```python
from build123d import *

# Parameters (mm, degrees)
BOSS_EXTRUDE1_DEPTH = 8
SKETCH12_W          = 1.5
SKETCH12_H          = 8.6
BOSS_EXTRUDE8_DEPTH = 3
BOSS_EXTRUDE5_DEPTH = 3
BOSS_EXTRUDE6_START = 8.75
SKETCH10_R          = 1.75
BOSS_EXTRUDE6_DEPTH = 8.75
SKETCH11_W          = 14.1
SKETCH11_H          = 1.5
BOSS_EXTRUDE7_DEPTH = 1.5
FILLET1_R           = 2
CUT_EXTRUDE2_REACH  = 69.432
SKETCH13_W          = 14
SKETCH13_H          = 7.25
FILLET2_R           = 1
SKETCH14_W          = 11
SKETCH14_H          = 52.76
CUT_EXTRUDE3_DEPTH  = 1
SKETCH15_W          = 5.5
SKETCH15_H          = 50.26
CUT_EXTRUDE4_DEPTH  = 1.5
SKETCH17_W          = 4
SKETCH17_H          = 5
SKETCH17_R          = 1
BOSS_EXTRUDE9_DEPTH = 1


with BuildPart() as part:
    # Sketch1 → Boss-Extrude1 (new body)
    with BuildSketch(Plane.XY):
        with BuildLine():
            Line((-0.5, 27.44), (-0.5, 0.5))
            ThreePointArc((-0.5, 0.5), (0.818019485, -2.681980515), (4, -4))
            Line((4, -4), (30.29, -4))
            ThreePointArc((30.29, -4), (33.471980515, -2.681980515), (34.79, 0.5))
            Line((34.79, 0.5), (34.79, 44.26))
            ThreePointArc((34.79, 44.26), (33.471980515, 47.441980515), (30.29, 48.76))
            Line((30.29, 48.76), (4, 48.76))
            ThreePointArc((4, 48.76), (0.818019485, 47.441980515), (-0.5, 44.26))
            Line((-0.5, 44.26), (-0.5, 36.04))
            Line((-0.5, 36.04), (-2, 36.04))
            Line((-2, 36.04), (-2, 44.26))
            ThreePointArc((-2, 44.26), (-0.242640687, 48.502640687), (4, 50.26))
            Line((4, 50.26), (30.29, 50.26))
            ThreePointArc((30.29, 50.26), (34.532640687, 48.502640687), (36.29, 44.26))
            Line((36.29, 44.26), (36.29, 0.5))
            ThreePointArc((36.29, 0.5), (34.532640687, -3.742640687), (30.29, -5.5))
            Line((30.29, -5.5), (4, -5.5))
            ThreePointArc((4, -5.5), (-0.242640687, -3.742640687), (-2, 0.5))
            Line((-2, 0.5), (-2, 27.44))
            Line((-2, 27.44), (-0.5, 27.44))
        make_face()
    extrude(amount=BOSS_EXTRUDE1_DEPTH)

    # Sketch12 → Boss-Extrude8 (add)
    with BuildSketch(Plane.XY.offset(8)):
        with Locations((-1.25, 31.74)):
            Rectangle(SKETCH12_W, SKETCH12_H)
    extrude(amount=-BOSS_EXTRUDE8_DEPTH)

    # Sketch8 → Boss-Extrude5 (add)
    with BuildSketch(Plane.XY.offset(8)):
        with BuildLine():
            Line((-2, 44.26), (-2, 0.5))
            ThreePointArc((-2, 0.5), (-0.242640687, -3.742640687), (4, -5.5))
            Line((4, -5.5), (30.29, -5.5))
            ThreePointArc((30.29, -5.5), (34.532640687, -3.742640687), (36.29, 0.5))
            Line((36.29, 0.5), (36.29, 44.26))
            ThreePointArc((36.29, 44.26), (34.532640687, 48.502640687), (30.29, 50.26))
            Line((30.29, 50.26), (4, 50.26))
            ThreePointArc((4, 50.26), (-0.242640687, 48.502640687), (-2, 44.26))
        make_face()
    extrude(amount=BOSS_EXTRUDE5_DEPTH)

    # Sketch10 → Boss-Extrude6 (add)
    # profile 1 of 4: a face of its own
    with BuildSketch(Plane(origin=(0, 0, 8), x_dir=(-1, 0, 0), z_dir=(0, 0, -1)).offset(BOSS_EXTRUDE6_START)):
        with BuildLine():
            Line((-30.29, 48.76), (-26.73, 48.76))
            Line((-26.73, 48.76), (-26.73, 44.45))
            ThreePointArc((-26.73, 44.45), (-27.828349571, 41.798349571), (-30.48, 40.7))
            Line((-30.48, 40.7), (-34.79, 40.7))
            Line((-34.79, 40.7), (-34.79, 44.26))
            ThreePointArc((-34.79, 44.26), (-33.471980515, 47.441980515), (-30.29, 48.76))
        make_face()
        with Locations(Location((-30.48, 44.45, 0), (0, 0, 180))):
            Circle(SKETCH10_R, mode=Mode.SUBTRACT)
    # profile 2 of 4: a face of its own
    with BuildSketch(Plane(origin=(0, 0, 8), x_dir=(-1, 0, 0), z_dir=(0, 0, -1)).offset(BOSS_EXTRUDE6_START)):
        with BuildLine():
            Line((-3.81, 40.7), (0.5, 40.7))
            Line((0.5, 40.7), (0.5, 44.26))
            ThreePointArc((0.5, 44.26), (-0.818019485, 47.441980515), (-4, 48.76))
            Line((-4, 48.76), (-7.56, 48.76))
            Line((-7.56, 48.76), (-7.56, 44.45))
            ThreePointArc((-7.56, 44.45), (-6.461650429, 41.798349571), (-3.81, 40.7))
        make_face()
        with Locations(Location((-3.81, 44.45, 0), (0, 0, 180))):
            Circle(SKETCH10_R, mode=Mode.SUBTRACT)
    # profile 3 of 4: a face of its own
    with BuildSketch(Plane(origin=(0, 0, 8), x_dir=(-1, 0, 0), z_dir=(0, 0, -1)).offset(BOSS_EXTRUDE6_START)):
        with BuildLine():
            Line((0.5, 7.56), (0.5, 0.5))
            ThreePointArc((0.5, 0.5), (-0.818019485, -2.681980515), (-4, -4))
            Line((-4, -4), (-7.56, -4))
            Line((-7.56, -4), (-7.56, 3.81))
            ThreePointArc((-7.56, 3.81), (-6.461650429, 6.461650429), (-3.81, 7.56))
            Line((-3.81, 7.56), (0.5, 7.56))
        make_face()
        with Locations(Location((-3.81, 3.81, 0), (0, 0, 180))):
            Circle(SKETCH10_R, mode=Mode.SUBTRACT)
    # profile 4 of 4: a face of its own
    with BuildSketch(Plane(origin=(0, 0, 8), x_dir=(-1, 0, 0), z_dir=(0, 0, -1)).offset(BOSS_EXTRUDE6_START)):
        with BuildLine():
            Line((-26.73, -4), (-30.29, -4))
            ThreePointArc((-30.29, -4), (-33.471980515, -2.681980515), (-34.79, 0.5))
            Line((-34.79, 0.5), (-34.79, 7.56))
            Line((-34.79, 7.56), (-30.48, 7.56))
            ThreePointArc((-30.48, 7.56), (-27.828349571, 6.461650429), (-26.73, 3.81))
            Line((-26.73, 3.81), (-26.73, -4))
        make_face()
        with Locations(Location((-30.48, 3.81, 0), (0, 0, 180))):
            Circle(SKETCH10_R, mode=Mode.SUBTRACT)
    extrude(amount=-BOSS_EXTRUDE6_DEPTH)

    # Sketch11 → Boss-Extrude7 (add)
    with BuildSketch(Plane(origin=(0, 0, 8), x_dir=(-1, 0, 0), z_dir=(0, 0, -1))):
        with Locations((-17.145, -4.75)):
            Rectangle(SKETCH11_W, SKETCH11_H)
    extrude(amount=BOSS_EXTRUDE7_DEPTH)

    # Fillet1
    fillet1_edges = [part.edges().sort_by_distance(p)[0] for p in [
        (17.145, -5.5, 11),
        (36.29, 22.38, 11),
        (34.532640687, 48.502640687, 11),
        (17.145, 50.26, 11),
        (-0.242640687, 48.502640687, 11),
        (-2, 22.38, 11),
        (-0.242640687, -3.742640687, 11),
        (34.532640687, -3.742640687, 11),
    ]]
    fillet(fillet1_edges, radius=FILLET1_R)

    # Sketch13 → Cut-Extrude2 (cut, up to next)
    with BuildSketch(Plane.XZ.offset(5.5), mode=Mode.PRIVATE) as cut_extrude2_sk1:
        with Locations((17.145, 3.625)):
            Rectangle(SKETCH13_W, SKETCH13_H)
    cut_extrude2_tool1 = extrude(cut_extrude2_sk1.sketch, amount=-CUT_EXTRUDE2_REACH, mode=Mode.PRIVATE) & part.part
    add(cut_extrude2_tool1.solids().sort_by_distance((17.145, -5.5, 3.625))[0], mode=Mode.SUBTRACT)

    # Fillet2
    fillet2_edges = [part.edges().sort_by_distance(p)[0] for p in [
        (-1.25, 36.04, 5),
        (-1.25, 27.44, 5),
        (10.145, -4.75, 7.25),
        (24.145, -4.75, 7.25),
    ]]
    fillet(fillet2_edges, radius=FILLET2_R)

    # Sketch14 → Cut-Extrude3 (cut)
    with BuildSketch(Plane(origin=(0, 0, 8), x_dir=(-1, 0, 0), z_dir=(0, 0, -1))):
        with Locations((-17.145, 22.38)):
            Rectangle(SKETCH14_W, SKETCH14_H)
    extrude(amount=-CUT_EXTRUDE3_DEPTH, mode=Mode.SUBTRACT)

    # Sketch15 → Cut-Extrude4 (cut)
    with BuildSketch(Plane(origin=(0, 0, 9), x_dir=(-1, 0, 0), z_dir=(0, 0, -1))):
        with Locations((-15.895, 22.38)):
            Rectangle(SKETCH15_W, SKETCH15_H)
    extrude(amount=-CUT_EXTRUDE4_DEPTH, mode=Mode.SUBTRACT)

    # Sketch17 → Boss-Extrude9 (add)
    # profile 1 of 2: a face of its own
    with BuildSketch(Plane(origin=(0, 0, 9), x_dir=(-1, 0, 0), z_dir=(0, 0, -1))):
        with Locations((-20.645, 9.86)):
            Rectangle(SKETCH17_W, SKETCH17_H)
        with Locations((-20.145, 9.86)):
            Circle(SKETCH17_R, mode=Mode.SUBTRACT)
    # profile 2 of 2: a face of its own
    with BuildSketch(Plane(origin=(0, 0, 9), x_dir=(-1, 0, 0), z_dir=(0, 0, -1))):
        with Locations((-20.645, 35.26)):
            Rectangle(SKETCH17_W, SKETCH17_H)
        with Locations((-20.145, 35.26)):
            Circle(SKETCH17_R, mode=Mode.SUBTRACT)
    extrude(amount=BOSS_EXTRUDE9_DEPTH)


solid = part.part
```
For this review, take the finished solid that the model builds, in its own axes (mm). A direction names the side the tool comes from. Round coordinates to 2 decimals unless told otherwise and drop trailing zeros. Write each loop counter-clockwise with the first axis right and the second up, starting at its lowest first coordinate (ties: lowest second). Pieces come first, ordered by that corner, then holes. Notation, with made-up numbers: (-7, 32) - (22, 32) arc R18 cw to (22, 46) - close; hole circle Ø1 at (26.5, 47.25). An arc over 180 degrees is marked (long way). Answer as a JSON object with one key per item and string values.
1. Tool access review of faces 1 (the face through (0.783, 47.407, -0.38)), 2 (the face through (31, 47, -0.75)), 3 (the face through (5, 23, 8)), 4 (the face through (0.783, -2.647, -0.38)), 5 (the face through (10.145, -5, 3)): name each direction out of +Z, -Z, +X, -X, +Y, -Y from which nothing blocks a thin tool from reaching the whole face with its end or side.
Response values:
{"face 1": "-Z, -X, +Y", "face 2": "-Z, +X, -X, +Y, -Y", "face 3": "-Z", "face 4": "-Z, -X, -Y", "face 5": "-Z, -Y"}
2. We need section A-A on y = 15. Give the boundary of the cut face in (x, z) (3 decimals), then the cut area to 3 significant figures.
Response values:
{"outline": "(-2, 0) - (-0.5, 0) - (-0.5, 8) - (11.645, 8) - (11.645, 9) - (13.145, 9) - (13.145, 10.5) - (18.645, 10.5) - (18.645, 9) - (22.645, 9) - (22.645, 8) - (34.79, 8) - (34.79, 0) - (36.29, 0) - (36.29, 9) arc R2 ccw to (34.29, 11) - (0, 11) arc R2 ccw to (-2, 9) - close", "area": "118 mm2"}
3. Draft analysis for pull direction X (two halves, no side actions). For faces 6 (the face through (-0.289, -3.696, 4.437)), 7 (the face through (-1, 32, 5)), 8 (the face through (-0.5, 20, 4)), state which applies: +X half, -X half, draft (parallel to the pull), parting line (faces both ways), or undercut.
Response values:
{"face 6": "-X half", "face 7": "draft", "face 8": "undercut"}
4. For pin 1 Ø6 at (x, y) = (17, 19.5) entering from -Z; pin 2 Ø2 at (y, z) = (45.5, 3.5) entering from -X; pin 3 Ø8 at (x, y) = (23, 27) entering from -Z, all flat-tipped, find the tip position at first contact; note any pin that passes through.
Response values:
{"pin 1": "stops at z = 9", "pin 2": "stops at x = -2", "pin 3": "stops at z = 8"}
5. To check wall thickness, follow line 1 along X through (y, z) = (44.45, 4); line 2 along Y through (x, z) = (30.48, 5.25); line 3 along Y through (x, z) = (26.5, 5.5). State the ranges of each line that lie inside material, in increasing order.
Response values:
{"line 1": "x = -2 to 2.06, 5.56 to 7.56, 26.73 to 28.73, 32.23 to 36.29", "line 2": "y = -5.5 to 2.06, 5.56 to 7.56, 40.7 to 42.7, 46.2 to 50.26", "line 3": "y = -5.5 to -4, 48.76 to 50.26"}
6. We need section B-B on z = 9.75. Give the boundary of the cut face in (x, y) (3 decimals), then the cut area to 3 significant figures.
Response values:
{"outline": "(-1.854, 0.5) arc R5.854 ccw to (4, -5.354) - (30.29, -5.354) arc R5.854 ccw to (36.144, 0.5) - (36.144, 44.26) arc R5.854 ccw to (30.29, 50.114) - (4, 50.114) arc R5.854 ccw to (-1.854, 44.26) - close; hole (13.145, -2.75) - (18.645, -2.75) - (18.645, 47.51) - (13.145, 47.51) - close", "area": "1,800 mm2"}
7. We need section C-C on x = 14. Give the boundary of the cut face in (y, z).
Response values:
{"outline": "(-5.5, 7.25) - (-4, 7.25) - (-4, 9) - (-2.75, 9) - (-2.75, 10.5) - (47.51, 10.5) - (47.51, 9) - (48.76, 9) - (48.76, 0) - (50.26, 0) - (50.26, 9) arc R2 ccw to (48.26, 11) - (-3.5, 11) arc R2 ccw to (-5.5, 9) - close"}
